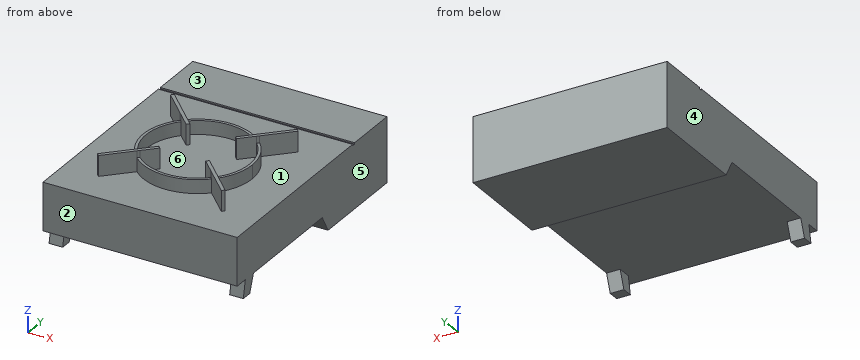
from build123d import *

# Parameters (mm, degrees)
F0_W      = 285
F0_H      = 370
F1_DEPTH  = 95
F2_W      = 285
F2_H      = 5
F3_DEPTH  = 2
F5_DEPTH  = 30
F6_DEPTH  = 20
F8_DEPTH  = 406
F9_W      = 245
F9_H      = 25
F10_DEPTH = 81


with BuildPart() as f1:
    # F0 (on Top) → F1 (new body)
    with BuildSketch(Plane.XY):
        with Locations((-142.5, 185)):
            Rectangle(F0_W, F0_H)
    extrude(amount=F1_DEPTH)

    # F2 (on face) → F3 (cut)
    with BuildSketch(Plane.XY.offset(95)):
        with Locations((-142.5, 287.5)):
            Rectangle(F2_W, F2_H)
    extrude(amount=-F3_DEPTH, mode=Mode.SUBTRACT)

    # F4 (on face) → F5 (join)
    with BuildSketch(Plane.XY.offset(95)):
        with BuildLine():
            Line((-232.6391152703, 48.8253508238), (-197.2731474365, 84.1913186575))
            ThreePointArc((-197.2731474365, 84.1913186575), (-199.0685424949, 85.9314575051), (-200.8086813425, 87.7268525635))
            Line((-200.8086813425, 87.7268525635), (-236.1746491762, 52.3608847297))
            Line((-236.1746491762, 52.3608847297), (-232.6391152703, 48.8253508238))
        make_face()
        with BuildLine():
            ThreePointArc((-200.8086813425, 87.7268525635), (-199.0685424949, 85.9314575051), (-197.2731474365, 84.1913186575))
            Line((-197.2731474365, 84.1913186575), (-194.4432654333, 87.0212006608))
            ThreePointArc((-194.4432654333, 87.0212006608), (-196.2401153702, 88.7598846298), (-197.9787993392, 90.5567345667))
            Line((-197.9787993392, 90.5567345667), (-200.8086813425, 87.7268525635))
        make_face()
        with BuildLine():
            ThreePointArc((-197.9787993392, 90.5567345667), (-196.2401153702, 88.7598846298), (-194.4432654333, 87.0212006608))
            Line((-194.4432654333, 87.0212006608), (-176.0875721064, 105.3768939877))
            Line((-176.0875721064, 105.3768939877), (-179.6231060123, 108.9124278936))
            Line((-179.6231060123, 108.9124278936), (-197.9787993392, 90.5567345667))
        make_face()
        with BuildLine():
            ThreePointArc((-90.5567345667, 87.0212006608), (-88.7598846298, 88.7598846298), (-87.0212006608, 90.5567345667))
            Line((-87.0212006608, 90.5567345667), (-105.3768939877, 108.9124278936))
            Line((-105.3768939877, 108.9124278936), (-108.9124278936, 105.3768939877))
            Line((-108.9124278936, 105.3768939877), (-90.5567345667, 87.0212006608))
        make_face()
        with BuildLine():
            ThreePointArc((-87.7268525635, 84.1913186575), (-85.9314575051, 85.9314575051), (-84.1913186575, 87.7268525635))
            Line((-84.1913186575, 87.7268525635), (-87.0212006608, 90.5567345667))
            ThreePointArc((-87.0212006608, 90.5567345667), (-88.7598846298, 88.7598846298), (-90.5567345667, 87.0212006608))
            Line((-90.5567345667, 87.0212006608), (-87.7268525635, 84.1913186575))
        make_face()
        with BuildLine():
            Line((-48.8253508238, 52.3608847297), (-84.1913186575, 87.7268525635))
            ThreePointArc((-84.1913186575, 87.7268525635), (-85.9314575051, 85.9314575051), (-87.7268525635, 84.1913186575))
            Line((-87.7268525635, 84.1913186575), (-52.3608847297, 48.8253508238))
            Line((-52.3608847297, 48.8253508238), (-48.8253508238, 52.3608847297))
        make_face()
        with BuildLine():
            ThreePointArc((-200.8086813425, 197.2731474365), (-199.0685424949, 199.0685424949), (-197.2731474365, 200.8086813425))
            Line((-197.2731474365, 200.8086813425), (-232.6391152703, 236.1746491762))
            Line((-232.6391152703, 236.1746491762), (-236.1746491762, 232.6391152703))
            Line((-236.1746491762, 232.6391152703), (-200.8086813425, 197.2731474365))
        make_face()
        with BuildLine():
            Line((-194.4432654333, 197.9787993392), (-197.2731474365, 200.8086813425))
            ThreePointArc((-197.2731474365, 200.8086813425), (-199.0685424949, 199.0685424949), (-200.8086813425, 197.2731474365))
            Line((-200.8086813425, 197.2731474365), (-197.9787993392, 194.4432654333))
            ThreePointArc((-197.9787993392, 194.4432654333), (-196.2401153702, 196.2401153702), (-194.4432654333, 197.9787993392))
        make_face()
        with BuildLine():
            Line((-176.0875721064, 179.6231060123), (-194.4432654333, 197.9787993392))
            ThreePointArc((-194.4432654333, 197.9787993392), (-196.2401153702, 196.2401153702), (-197.9787993392, 194.4432654333))
            Line((-197.9787993392, 194.4432654333), (-179.6231060123, 176.0875721064))
            Line((-179.6231060123, 176.0875721064), (-176.0875721064, 179.6231060123))
        make_face()
        with BuildLine():
            ThreePointArc((-87.7268525635, 200.8086813425), (-85.9314575051, 199.0685424949), (-84.1913186575, 197.2731474365))
            Line((-84.1913186575, 197.2731474365), (-48.8253508238, 232.6391152703))
            Line((-48.8253508238, 232.6391152703), (-52.3608847297, 236.1746491762))
            Line((-52.3608847297, 236.1746491762), (-87.7268525635, 200.8086813425))
        make_face()
        with BuildLine():
            Line((-87.0212006608, 194.4432654333), (-84.1913186575, 197.2731474365))
            ThreePointArc((-84.1913186575, 197.2731474365), (-85.9314575051, 199.0685424949), (-87.7268525635, 200.8086813425))
            Line((-87.7268525635, 200.8086813425), (-90.5567345667, 197.9787993392))
            ThreePointArc((-90.5567345667, 197.9787993392), (-88.7598846298, 196.2401153702), (-87.0212006608, 194.4432654333))
        make_face()
        with BuildLine():
            Line((-105.3768939877, 176.0875721064), (-87.0212006608, 194.4432654333))
            ThreePointArc((-87.0212006608, 194.4432654333), (-88.7598846298, 196.2401153702), (-90.5567345667, 197.9787993392))
            Line((-90.5567345667, 197.9787993392), (-108.9124278936, 179.6231060123))
            Line((-108.9124278936, 179.6231060123), (-105.3768939877, 176.0875721064))
        make_face()
    extrude(amount=F5_DEPTH)

    # F4 (on face) → F6 (join)
    with BuildSketch(Plane.XY.offset(95)):
        with BuildLine():
            ThreePointArc((-197.2731474365, 84.1913186575), (-142.5, 62.5), (-87.7268525635, 84.1913186575))
            Line((-87.7268525635, 84.1913186575), (-90.5567345667, 87.0212006608))
            ThreePointArc((-90.5567345667, 87.0212006608), (-142.5, 66.5), (-194.4432654333, 87.0212006608))
            Line((-194.4432654333, 87.0212006608), (-197.2731474365, 84.1913186575))
        make_face()
        with BuildLine():
            Line((-197.9787993392, 194.4432654333), (-200.8086813425, 197.2731474365))
            ThreePointArc((-200.8086813425, 197.2731474365), (-222.5, 142.5), (-200.8086813425, 87.7268525635))
            Line((-200.8086813425, 87.7268525635), (-197.9787993392, 90.5567345667))
            ThreePointArc((-197.9787993392, 90.5567345667), (-218.5, 142.5), (-197.9787993392, 194.4432654333))
        make_face()
        with BuildLine():
            Line((-90.5567345667, 197.9787993392), (-87.7268525635, 200.8086813425))
            ThreePointArc((-87.7268525635, 200.8086813425), (-142.5, 222.5), (-197.2731474365, 200.8086813425))
            Line((-197.2731474365, 200.8086813425), (-194.4432654333, 197.9787993392))
            ThreePointArc((-194.4432654333, 197.9787993392), (-142.5, 218.5), (-90.5567345667, 197.9787993392))
        make_face()
        with BuildLine():
            ThreePointArc((-84.1913186575, 87.7268525635), (-68.1202497067, 113.0440541435), (-62.5, 142.5))
            ThreePointArc((-62.5, 142.5), (-68.1202497067, 171.9559458565), (-84.1913186575, 197.2731474365))
            Line((-84.1913186575, 197.2731474365), (-87.0212006608, 194.4432654333))
            ThreePointArc((-87.0212006608, 194.4432654333), (-71.8162368369, 170.4250000019), (-66.5, 142.5))
            ThreePointArc((-66.5, 142.5), (-71.8162368369, 114.5749999981), (-87.0212006608, 90.5567345667))
            Line((-87.0212006608, 90.5567345667), (-84.1913186575, 87.7268525635))
        make_face()
    extrude(amount=F6_DEPTH)

    # F7 (on face) → F8 (cut)
    with BuildSketch(Plane.YZ):
        Polygon((0, 0), (15, 0), (20, 25), (0, 25), align=None)
        Polygon((40, 25), (30.9007441433, 0), (224.4337567297, 0), (210, 25), align=None)
    extrude(amount=-F8_DEPTH, mode=Mode.SUBTRACT)

    # F9 (on face) → F10 (cut)
    with BuildSketch(Plane.XZ):
        with Locations((-142.5, 12.5)):
            Rectangle(F9_W, F9_H)
    extrude(amount=-F10_DEPTH, mode=Mode.SUBTRACT)


solid = f1.part
Here's how the part is built. I have some questions about the finished solid (model axes, mm). Face numbers are marked on the shaded views. A direction names the side the tool comes from. Coordinates: 2 decimals unless noted, no trailing zeros. Loops run counter-clockwise (first coordinate to the right, second up) from the corner with the lowest first, then second, coordinate; pieces in that order, holes last. Notation, with made-up numbers: (-0.75, 60) -> (26.25, 60) arc R20 cw to (26.25, 83) -> close; hole circle Ø1 at (-18.75, -10). An arc over 180 degrees is marked (long way). Use one line per item in the form item = value. Start each with the question number.
(1) On a 3-axis mill with a long thin cutter (end or side, diameter ignored), from which of +Z, -Z, +X, -X, +Y, -Y can I reach the whole of each face in a straight line? I mean the marked faces 1 and 2. Say none if no direction works.
(2) Will these pins go through, and if not, where does the flat tip stop? pin 1 (5 mm diameter, centred on x = -37.5, y = 162, fed in from -Z); pin 2 (19.5 mm diameter, centred on x = -205.5, y = 131.5, fed in from +Z); pin 3 (1.6 mm diameter, centred on x = -172.5, z = 93.5, fed in from -Y); pin 4 (1.5 mm diameter, centred on x = -95.5, y = 287.5, fed in from +Z).
(3) If we section it at A-A (z = 12): Please give me the cut outline in (x, y).
(4) If we section it at C-C (x = -36.5): Please give me the cut outline in (y, z).
(5) We'd pull the mould along X, two halves only. Please class the marked faces 3, 4, 5 and 6: pulls with the +X half, pulls with the -X half, needs draft (parallel to the pull), parting line crosses it, or undercut.
(6) Please list where these lines run through material, in increasing order: line 1 along Z through (x, y) = (-154, 31.5); line 2 along Z through (x, y) = (-94, 347.5); line 3 along Y through (x, z) = (-164.5, 111.5).
(7) If we section it at D-D (y = 96.5): Please give me the cut outline in (x, z), then the cut area to 3 significant figures.
Verdict:
q1.face_1 = +Z
q1.face_2 = +Z, -Z, +X, -X, -Y
q2.pin_1 = 25
q2.pin_2 = 95
q2.pin_3 = 0
q2.pin_4 = 93
q3.outline = (-285, 17.4) -> (-265, 17.4) -> (-265, 35.27) -> (-285, 35.27) -> close; (-285, 217.51) -> (0, 217.51) -> (0, 370) -> (-285, 370) -> close; (-20, 17.4) -> (0, 17.4) -> (0, 35.27) -> (-20, 35.27) -> close
q4.outline = (0, 25) -> (210, 25) -> (224.43, 0) -> (370, 0) -> (370, 95) -> (290, 95) -> (290, 93) -> (285, 93) -> (285, 95) -> (0, 95) -> close
q5.face_3 = needs draft
q5.face_4 = pulls with the -X half
q5.face_5 = pulls with the +X half
q5.face_6 = undercut
q6.line_1 = 25 to 95
q6.line_2 = 0 to 95
q6.line_3 = 65.58 to 69.75, 215.25 to 219.42
q7.outline = (-285, 25) -> (0, 25) -> (0, 95) -> (-77.05, 95) -> (-77.05, 115) -> (-82, 115) -> (-82, 95) -> (-92.96, 95) -> (-92.96, 125) -> (-100.04, 125) -> (-100.04, 95) -> (-184.96, 95) -> (-184.96, 125) -> (-192.04, 125) -> (-192.04, 95) -> (-203, 95) -> (-203, 115) -> (-207.95, 115) -> (-207.95, 95) -> (-285, 95) -> close
q7.area = 20,600 mm²
